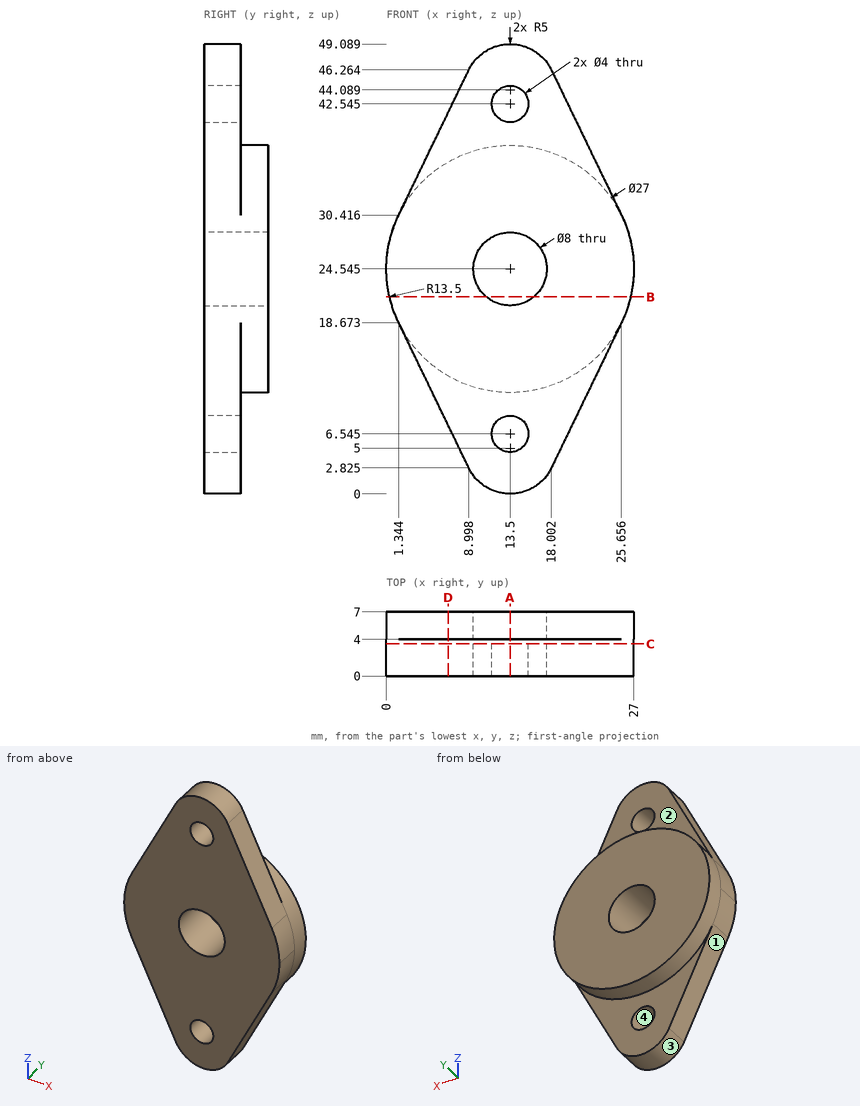
Source: three-view drawing plus pictorial views. Frame: mm from the lowest corner of the part. Coordinates: 2 decimals unless noted, no trailing zeros. Order: outer loops, then holes, each group sorted by start corner. A loop starts at its lowest first (then second) coordinate and runs counter-clockwise, first axis right, second up.
Item 1: Cut plane A-A (x = 13.5). Return loops of the section in (y, z) (1 decimal), plus the area to 3 significant figures.
Output values:
outline: (0, 0) - (4, 0) - (4, 4.5) - (0, 4.5) - close; (0, 8.5) - (4, 8.5) - (4, 11) - (7, 11) - (7, 20.5) - (0, 20.5) - close; (0, 28.5) - (7, 28.5) - (7, 38) - (4, 38) - (4, 40.5) - (0, 40.5) - close; (0, 44.5) - (4, 44.5) - (4, 49.1) - (0, 49.1) - close
area: 189 mm2
Item 2: Cut plane C-C (y = 3.5). Return loops of the section in (x, z) (1 decimal), plus the area to 3 significant figures.
Output values:
outline: (1.3, 18.7) - (9, 2.8) arc R5 ccw to (18, 2.8) - (25.7, 18.7) arc R13.5 ccw to (25.7, 30.4) - (18, 46.3) arc R5 ccw to (9, 46.3) - (1.3, 30.4) arc R13.5 ccw to start; hole circle Ø8 at (13.5, 24.5); hole circle Ø4 at (13.5, 6.5); hole circle Ø4 at (13.5, 42.5)
area: 796 mm2
Item 3: Cut plane D-D (x = 6.75). Return loops of the section in (y, z) (1 decimal).
Output values:
outline: (0, 7.5) - (4, 7.5) - (4, 12.9) - (7, 12.9) - (7, 36.2) - (4, 36.2) - (4, 41.6) - (0, 41.6) - close
Item 4: Material intervals for line 1 (Y direction, x = 11, z = 5); line 2 (X direction, y = 5.5, z = 25) (1 decimal); line 3 (X direction, y = 2.75, z = 43.5) (1 decimal), sorted ascending.
Output values:
line 1: y = 0 to 4
line 2: x = 0 to 9.5, 17.5 to 27
line 3: x = 7.7 to 11.7, 15.3 to 19.3
Item 5: Cut plane B-B (z = 21.5). Return loops of the section in (x, y) (1 decimal).
Output values:
outline: (0.3, 0) - (10.9, 0) - (10.9, 7) - (0.3, 7) - close; (16.1, 0) - (26.7, 0) - (26.7, 7) - (16.1, 7) - close
Item 6: First-contact query: P1, Ø3, axis at x = 9, y = 3.5, coming from the -Z side; P2, Ø2.5, axis at x = 13.5, z = 6.54, coming from the -Y side; P3, Ø2, axis at y = 4, z = 17.5, coming from the +X side; P4, Ø6.5, axis at x = 13.5, z = 42.54, coming from the +Y side. Flat tips, straight axial feed; report the tip coordinate or a pass-through.
Output values:
P1: stops at z = 1
P2: passes through
P3: stops at x = 25.57
P4: stops at y = 4
Item 7: Pull-direction query (X, two-part tool) for the marked faces 1, 2, 3 and 4; classes: pulls with the +X half, pulls with the -X half, needs draft (parallel to the pull), parting line crosses it, or undercut.
Output values:
face 1: pulls with the -X half
face 2: needs draft
face 3: parting line crosses it
face 4: undercut
